from build123d import *

# Parameters (mm, degrees)
SKETCH1_W           = 358
SKETCH1_H           = 120
BOSS_EXTRUDE1_DEPTH = 3
SKETCH2_R           = 15
SKETCH2_R_2         = 9
CUT_EXTRUDE1_DEPTH  = 10
SKETCH3_R           = 3.1
SKETCH3_R_2         = 4
SKETCH3_R_3         = 5
CUT_EXTRUDE2_DEPTH  = 10
CUT_EXTRUDE3_DEPTH  = 10


with BuildPart() as part:
    # Sketch1 → Boss-Extrude1 (new body)
    with BuildSketch(Plane.XY):
        Rectangle(SKETCH1_W, SKETCH1_H)
    extrude(amount=BOSS_EXTRUDE1_DEPTH)

    # Sketch2 → Cut-Extrude1 (cut)
    with BuildSketch(Plane.XY.offset(3)):
        with Locations((129, 0)):
            Circle(SKETCH2_R)
        with Locations((83.17424305, 20)):
            Circle(SKETCH2_R_2)
        with Locations((82.45294449, -18.261544956)):
            Circle(SKETCH2_R_2)
    extrude(amount=-CUT_EXTRUDE1_DEPTH, mode=Mode.SUBTRACT)

    # Sketch3 → Cut-Extrude2 (cut)
    with BuildSketch(Plane.XY.offset(3)):
        with Locations((-139, 33)):
            Circle(SKETCH3_R)
        with Locations((-139, 3)):
            Circle(SKETCH3_R_2)
        with Locations((-139, -27)):
            Circle(SKETCH3_R_3)
    extrude(amount=-CUT_EXTRUDE2_DEPTH, mode=Mode.SUBTRACT)

    # Sketch4 → Cut-Extrude3 (cut)
    with BuildSketch(Plane.XY.offset(3)):
        with BuildLine():
            Line((-159, -60), (-159, -47))
            ThreePointArc((-159, -47), (-156, -44), (-153, -47))
            Line((-153, -47), (-153, -60))
            Line((-153, -60), (-159, -60))
        make_face()
        with BuildLine():
            Line((-153, 47), (-153, 60))
            Line((-153, 60), (-159, 60))
            Line((-159, 60), (-159, 47))
            ThreePointArc((-159, 47), (-156, 44), (-153, 47))
        make_face()
        with BuildLine():
            Line((159, 60), (159, 47))
            ThreePointArc((159, 47), (156, 44), (153, 47))
            Line((153, 47), (153, 60))
            Line((153, 60), (159, 60))
        make_face()
        with BuildLine():
            Line((153, -47), (153, -60))
            Line((153, -60), (159, -60))
            Line((159, -60), (159, -47))
            ThreePointArc((159, -47), (156, -44), (153, -47))
        make_face()
        with BuildLine():
            Line((-179, 3), (-166, 3))
            ThreePointArc((-166, 3), (-163, 0), (-166, -3))
            Line((-166, -3), (-179, -3))
            Line((-179, -3), (-179, 3))
        make_face()
        with BuildLine():
            Line((-3, -60), (-3, -47))
            ThreePointArc((-3, -47), (0, -44), (3, -47))
            Line((3, -47), (3, -60))
            Line((3, -60), (-3, -60))
        make_face()
        with BuildLine():
            Line((166, -3), (179, -3))
            Line((179, -3), (179, 3))
            Line((179, 3), (166, 3))
            ThreePointArc((166, 3), (163, 0), (166, -3))
        make_face()
        with BuildLine():
            Line((3, 47), (3, 60))
            Line((3, 60), (-3, 60))
            Line((-3, 60), (-3, 47))
            ThreePointArc((-3, 47), (0, 44), (3, 47))
        make_face()
    extrude(amount=-CUT_EXTRUDE3_DEPTH, mode=Mode.SUBTRACT)


solid = part.part
CAD build for the part. Positions are in the model's coordinates, mm. Round coordinates to 2 decimals unless told otherwise and drop trailing zeros. Order: outer loops, then holes, each group sorted by start corner. A loop starts at its lowest first (then second) coordinate and runs counter-clockwise, first axis right, second up. Notation, with made-up numbers: (34.25, 9.25) -> (68.25, 9.25) arc R7 ccw to (68.25, 17.25) -> close; hole circle Ø4 at (27, 53.25). An arc over 180 degrees is marked (long way). Write each question's results on one line, items separated by ' | '.
1. Cut at A-A (x = -139). Give the cut face in (y, z), plus the area to 3 significant figures.
Findings below:
outline: (-60, 0) -> (-32, 0) -> (-32, 3) -> (-60, 3) -> close; (-22, 0) -> (-1, 0) -> (-1, 3) -> (-22, 3) -> close; (7, 0) -> (29.9, 0) -> (29.9, 3) -> (7, 3) -> close; (36.1, 0) -> (60, 0) -> (60, 3) -> (36.1, 3) -> close | area: 287 mm²
2. Flat gauge pin, fed straight in: P1, Ø5, axis at x = -115.5, y = 19.5, coming from the -Z side. Where does the tip first touch, or does it go through?
Findings below:
P1: stops at z = 0
3. Cut at B-B (x = 129). Give the cut face in (y, z), plus the area to 3 significant figures.
Findings below:
outline: (-60, 0) -> (-15, 0) -> (-15, 3) -> (-60, 3) -> close; (15, 0) -> (60, 0) -> (60, 3) -> (15, 3) -> close | area: 270 mm²
4. Wall check: line 1 along Y through (x, z) = (-139, 2); line 2 along X through (y, z) = (-52, 2.1); line 3 along Y through (x, z) = (127.5, 0.5). Give the ranges that are in metal, low to high. Write a range as [from, to].
Findings below:
line 1: y = [-60, -32], [-22, -1], [7, 29.9], [36.1, 60] | line 2: x = [-179, -159], [-153, -3], [3, 153], [159, 179] | line 3: y = [-60, -14.92], [14.92, 60]
5. Pull direction Y, two halves, no side cores. Call faces 1 (the face through (-136.043, 33.931, 1.521)), 2 (the face through (-3, 1, 0)): pulls with the +Y half, pulls with the -Y half, needs draft (parallel to the pull), parting line crosses it, or undercut.
Findings below:
face 1: undercut | face 2: needs draft
6. Cut at C-C (z = 1.2). Count the separate pieces of the cut face and the enclosed holes in it, plus the area to 3 significant figures.
Findings below:
separate pieces: 1 | enclosed holes: 6 | area: 40,800 mm²
